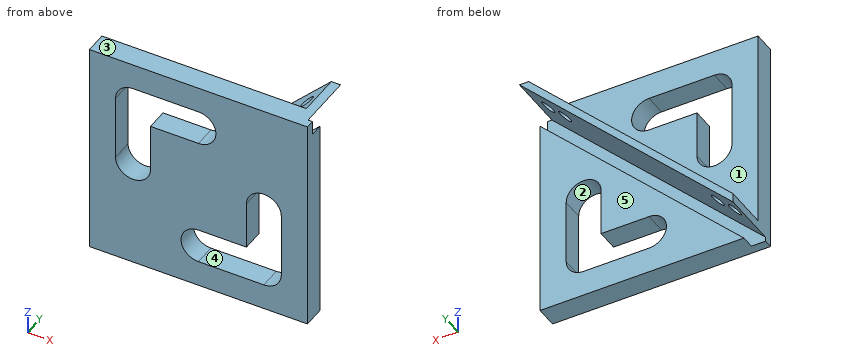
from build123d import *

# Parameters (mm, degrees)
SKETCH1_W           = 50
SKETCH1_H           = 50
BOSS_EXTRUDE1_DEPTH = 5
BOSS_EXTRUDE2_DEPTH = 10
CUT_EXTRUDE1_DEPTH  = 3
SKETCH4_R           = 1.65
CUT_EXTRUDE2_DEPTH  = 38.562445841


with BuildPart() as part:
    # Sketch1 → Boss-Extrude1 (new body)
    with BuildSketch(Plane(origin=(0, 0, 0), x_dir=(1, 0, 0), z_dir=(0, 1, 0))):
        Rectangle(SKETCH1_W, SKETCH1_H)
        with BuildLine():
            Line((15, 19), (0, 19))
            ThreePointArc((0, 19), (-4, 15), (0, 11))
            Line((0, 11), (11, 11))
            Line((11, 11), (11, 0))
            ThreePointArc((11, 0), (15, -4), (19, 0))
            Line((19, 0), (19, 15))
            ThreePointArc((19, 15), (17.828427125, 17.828427125), (15, 19))
        make_face(mode=Mode.SUBTRACT)
        with BuildLine():
            Line((-15, -19), (0, -19))
            ThreePointArc((0, -19), (4, -15), (0, -11))
            Line((0, -11), (-11, -11))
            Line((-11, -11), (-11, 0))
            ThreePointArc((-11, 0), (-15, 4), (-19, 0))
            Line((-19, 0), (-19, -15))
            ThreePointArc((-19, -15), (-17.828427125, -17.828427125), (-15, -19))
        make_face(mode=Mode.SUBTRACT)
    extrude(amount=BOSS_EXTRUDE1_DEPTH)

    # Sketch2 → Boss-Extrude2 (add)
    with BuildSketch(Plane(origin=(0, 5, 0), x_dir=(1, 0, 0), z_dir=(0, 1, 0))):
        Polygon((-25, 21.878679656), (21.878679656, -25), (24, -25), (-25, 24), align=None)
    extrude(amount=BOSS_EXTRUDE2_DEPTH)

    # Sketch3 → Cut-Extrude1 (cut)
    with BuildSketch(Plane(origin=(0, 5, 0), x_dir=(1, 0, 0), z_dir=(0, 1, 0))):
        Polygon((-21.757359313, 25), (25, -21.757359313), (25, -25), (24, -25), (-25, 24), (-25, 25), align=None)
    extrude(amount=-CUT_EXTRUDE1_DEPTH, mode=Mode.SUBTRACT)

    # Sketch4 → Cut-Extrude2 (cut, through all)
    with BuildSketch(Plane(origin=(-1.560660172, 0, 1.560660172), x_dir=(0.707106781, 0, 0.707106781), z_dir=(-0.707106781, 0, 0.707106781))):
        with Locations((-31.148232278, 10)):
            Circle(SKETCH4_R)
        with Locations((23.851767722, 10)):
            Circle(SKETCH4_R)
        with Locations((29.351767722, 10)):
            Circle(SKETCH4_R)
        with Locations((-25.648232278, 10)):
            Circle(SKETCH4_R)
    extrude(amount=-CUT_EXTRUDE2_DEPTH, mode=Mode.SUBTRACT)


solid = part.part
CAD build for the part. Positions are in the model's coordinates, mm. Face numbers are marked on the shaded views. A direction names the side the tool comes from. Round coordinates to 2 decimals unless told otherwise and drop trailing zeros. Order: outer loops, then holes, each group sorted by start corner. A loop starts at its lowest first (then second) coordinate and runs counter-clockwise, first axis right, second up. Notation, with made-up numbers: M 75,45 L 124,45 A21 ccw 124,50 Z; hole C 54.25,-7.5 d5. An arc over 180 degrees is marked long. Use one line per item in the form item = value.
Q1. Flat gauge pins, fed straight in: P1, Ø8, axis at y = 9.5, z = 17.5, coming from the -X side; P2, Ø3, axis at y = 11.5, z = -19, coming from the +X side; P3, Ø1.5, axis at x = -3, y = 10.5, coming from the +Z side. Where does each tip first touch, or does it go through?
Recorded:
P1 = 10.38
P2 = -18.51
P3 = 0.87
Q2. Saw through at B-B on x = -8.5. Give the cut face in (y, z).
Recorded:
outline = M 0,-25 L 5,-25 L 5,-11.74 L 2,-11.74 L 2,-7.5 L 15,-7.5 L 15,-5.38 L 5,-5.38 L 5,11 L 0,11 Z; M 0,19 L 5,19 L 5,25 L 0,25 Z
Q3. Saw through at A-A on y = 4. Give the cut face in (x, z), then the cut area to 3 significant figures.
Recorded:
outline = M -25,-24 L 24,25 L -25,25 Z; M -21.76,-25 L 25,-25 L 25,21.76 Z; hole M -19,0 A4 ccw -11,0 L -11,11 L 0,11 A4 ccw 0,19 L -15,19 A4 ccw -19,15 Z; hole M 0,-19 L 15,-19 A4 ccw 19,-15 L 19,0 A4 ccw 11,0 L 11,-11 L 0,-11 A4 ccw Z
area = 1,720 mm^2
Q4. Probe L1, parallel to Z at x = -7, y = 2.75; L2, parallel to Z at x = -7, y = 1; L3, parallel to X at y = 0.5, z = -0.5. List the from-to ranges inside material, lowest first.
Recorded:
L1 = -25 to -10.24, -6 to 11, 19 to 25
L2 = -25 to 11, 19 to 25
L3 = -25 to -18.97, -11.03 to 11, 19 to 25
Q5. Two-plate mould, pull along X, no slides. Class the marked faces 1 and 2: +X half, -X half, draft (parallel to the pull), parting line (faces both ways), or undercut.
Recorded:
face_1 = draft
face_2 = undercut
Q6. Which spindle directions (+Z, -Z, +X, -X, +Y, -Y) get a long thin tool onto all of the face, cutting with end or side? Do the marked faces 3, 4 and 5. Say none if no direction does.
Recorded:
face_3 = +Z, +X, -X, +Y, -Y
face_4 = +Y, -Y
face_5 = -Z, +X, +Y
